For this review, take the finished solid that the model builds, in its own axes (mm). A direction names the side the tool comes from. Give positions to 0.01 mm unless a question says otherwise; leave off trailing zeros. Write each loop counter-clockwise with the first axis right and the second up, starting at its lowest first coordinate (ties: lowest second). Pieces come first, ordered by that corner, then holes.
Q1. We need section C-C (z = -4.5). Write out the cut boundary in (x, y), then the cut area to 3 significant figures.
Q2. Machinability: for faces 4 (the flat face through (0, 0, 20)), 5 (the flat face through (1, -3, 10)), 6 (the flat face through (0, 0, -39)), which of the approach directions +Z, -Z, +X, -X, +Y, -Y give a long, thin tool a straight path to every point of the face, cutting with its end or side? Answer none if there is none.
Q3. Insertion check: P1, Ø2, axis at x = 12.99, y = -7.5, coming from the +Z side; P2, Ø1.5, axis at y = -4.5, z = 7.5, coming from the -X side; P3, Ø3, axis at x = 0, y = 15, coming from the +Z side; P4, Ø12, axis at y = 13.5, z = -29, coming from the -X side. Each pin has a flat end and moves straight along its axis. Give the tip position at first contact, or say it passes through.
Q4. For line 1 (Z direction, x = 5.5, y = 3.5); line 2 (Y direction, x = 0, z = -1.75); line 3 (X direction, y = 15, z = -3.75), list the stretches that pass through material, from the lowest coordinate up.
Q5. We need section A-A (y = 0). Write out the cut boundary in (x, z).
Q6. We need section D-D (x = 18). Write out the cut boundary in (y, z), then the cut area to 3 significant figures.
Q7. Mouldability with a two-part tool opening along Z and no side actions: class faces 1 (the conical face through (-0.064, 14.712, -7.844)), 2 (the cylindrical face through (6.466, -2.681, 20.846)), 3 (the flat face through (2.1, 2.4, 5)) as released by +Z, released by -Z, zero draft, split by the parting line, or undercut.
Q8. We need section B-B (z = 17.5). Write out the cut boundary in (x, y).
```python
from build123d import *

# Parameters (mm, degrees)
SKETCH1_R                = 20
BOSS_EXTRUDE1_DEPTH      = 39
SKETCH2_R                = 10
BOSS_EXTRUDE2_DEPTH      = 5
SKETCH7_R                = 3
BOSS_EXTRUDE3_DEPTH      = 5
BOSS_EXTRUDE4_DEPTH      = 10
M3_CLEARANCE_HOLE2_D     = 3.4
M3_CLEARANCE_HOLE2_DEPTH = 7
M3_CLEARANCE_HOLE2_TIP   = 1.021463052
SKETCH15_R               = 7
BOSS_EXTRUDE9_DEPTH      = 22
CUT_EXTRUDE3_START       = -12
SKETCH18_R               = 3
CUT_EXTRUDE3_DEPTH       = 12


with BuildPart() as part:
    # Sketch1 → Boss-Extrude1 (new body)
    with BuildSketch(Plane.XY):
        Circle(SKETCH1_R)
    extrude(amount=-BOSS_EXTRUDE1_DEPTH)

    # Sketch2 → Boss-Extrude2 (add)
    with BuildSketch(Plane.XY):
        Circle(SKETCH2_R)
    extrude(amount=BOSS_EXTRUDE2_DEPTH)

    # Sketch7 → Boss-Extrude3 (add)
    with BuildSketch(Plane.XY.offset(5)):
        Circle(SKETCH7_R)
    extrude(amount=BOSS_EXTRUDE3_DEPTH)

    # Sketch9 → Boss-Extrude4 (add)
    with BuildSketch(Plane.XY.offset(10)):
        with BuildLine():
            Line((-2.236067977, 2), (2.236067977, 2))
            ThreePointArc((2.236067977, 2), (0, -3), (-2.236067977, 2))
        make_face()
    extrude(amount=BOSS_EXTRUDE4_DEPTH)

    # M3 Clearance Hole2
    with Locations(Plane.XY):
        with Locations((0, 15), (12.991881057, -7.499133975), (-12.988881057, -7.500866025)):
            Hole(M3_CLEARANCE_HOLE2_D / 2, depth=M3_CLEARANCE_HOLE2_DEPTH)
            with Locations((0, 0, -(M3_CLEARANCE_HOLE2_DEPTH + M3_CLEARANCE_HOLE2_TIP / 2))):  # 118° drill point
                Cone(0, M3_CLEARANCE_HOLE2_D / 2, M3_CLEARANCE_HOLE2_TIP, mode=Mode.SUBTRACT)

    # Sketch15 → Boss-Extrude9 (add)
    with BuildSketch(Plane.XY.offset(10)):
        Circle(SKETCH15_R)
        with BuildLine():
            Line((-2.236067977, 2), (2.236067977, 2))
            ThreePointArc((2.236067977, 2), (0, -3), (-2.236067977, 2))
        make_face(mode=Mode.SUBTRACT)
    extrude(amount=BOSS_EXTRUDE9_DEPTH)

    # Sketch18 → Cut-Extrude3 (cut)
    with BuildSketch(Plane.XY.offset(32).offset(CUT_EXTRUDE3_START)):
        Circle(SKETCH18_R)
    extrude(amount=CUT_EXTRUDE3_DEPTH, mode=Mode.SUBTRACT)


solid = part.part
```
Computed:
1. outline: circle Ø40 at (0, 0); hole circle Ø3.4 at (-12.99, -7.5); hole circle Ø3.4 at (0, 15); hole circle Ø3.4 at (12.99, -7.5)
1. area: 1,230 mm2
2. face 4: +Z
2. face 5: none
2. face 6: -Z, +X, -X, +Y, -Y
3. P1: stops at z = -7.42
3. P2: passes through
3. P3: stops at z = -7.12
3. P4: stops at x = -18.54
4. line 1: z = -39 to 5, 10 to 32
4. line 2: y = -20 to 13.3, 16.7 to 20
4. line 3: x = -13.23 to -1.7, 1.7 to 13.23
5. outline: (-20, -39) - (20, -39) - (20, 0) - (10, 0) - (10, 5) - (3, 5) - (3, 10) - (7, 10) - (7, 32) - (3, 32) - (3, 20) - (-3, 20) - (-3, 32) - (-7, 32) - (-7, 10) - (-3, 10) - (-3, 5) - (-10, 5) - (-10, 0) - (-20, 0) - close
6. outline: (-8.72, -39) - (8.72, -39) - (8.72, 0) - (-8.72, 0) - close
6. area: 680 mm2
7. face 1: released by +Z
7. face 2: zero draft
7. face 3: undercut
8. outline: circle Ø14 at (0, 0)
